Input: dimensioned drawing with shaded views. Units: mm. Origin: part minimum x, y, z. A direction names the side the tool comes from. Round coordinates to 2 decimals unless told otherwise and drop trailing zeros. Loops run counter-clockwise (first coordinate to the right, second up) from the corner with the lowest first, then second, coordinate; pieces in that order, holes last. Notation, with made-up numbers: (3, 64.25) - (36, 64.25) arc R14 cw to (36, 89.25) - close; hole circle Ø8 at (58, 24.25). An arc over 180 degrees is marked (long way). Answer as CSV lines item,"result".
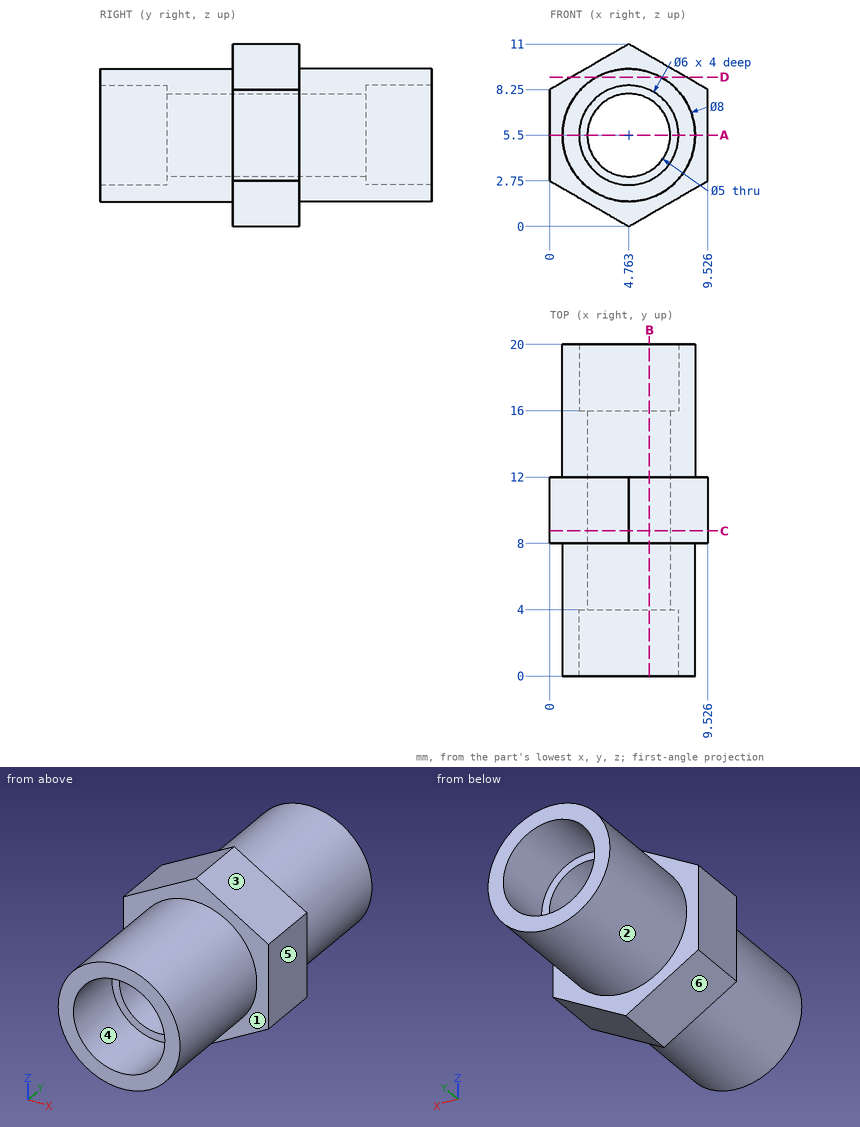
(1) Section A-A (z = 5.5). Output: boundary loops of the cut face in (x, y).
Findings below:
outline,"(0, 8) - (0.76, 8) - (0.76, 0) - (1.76, 0) - (1.76, 4) - (2.26, 4) - (2.26, 16) - (1.76, 16) - (1.76, 20) - (0.76, 20) - (0.76, 12) - (0, 12) - close; (7.26, 4) - (7.76, 4) - (7.76, 0) - (8.76, 0) - (8.76, 8) - (9.53, 8) - (9.53, 12) - (8.76, 12) - (8.76, 20) - (7.76, 20) - (7.76, 16) - (7.26, 16) - close"
(2) Section D-D (z = 9). Output: boundary loops of the cut face in (x, y).
Findings below:
outline,"(1.3, 8) - (2.83, 8) - (2.83, 0) - (6.7, 0) - (6.7, 8) - (8.23, 8) - (8.23, 12) - (6.7, 12) - (6.7, 20) - (2.83, 20) - (2.83, 12) - (1.3, 12) - close"
(3) Section C-C (y = 8.75). Output: boundary loops of the cut face in (x, z).
Findings below:
outline,"(0, 2.75) - (4.76, 0) - (9.53, 2.75) - (9.53, 8.25) - (4.76, 11) - (0, 8.25) - close; hole circle Ø5 at (4.76, 5.5)"
(4) Draft query along Z for the marked faces 4, 5 and 6. Return one class per face: pulls with the +Z half, pulls with the -Z half, needs draft (parallel to the pull), parting line crosses it, or undercut.
Findings below:
face 4,"undercut"
face 5,"needs draft"
face 6,"pulls with the -Z half"
(5) Material intervals for line 1 along X through (y, z) = (17.2, 5.5); line 2 along Z through (x, y) = (7, 4.5) (1 decimal); line 3 along X through (y, z) = (18.25, 2.75) (1 decimal), sorted ascending.
Findings below:
line 1,"0.76 to 1.76, 7.76 to 8.76"
line 2,"2.2 to 4.4, 6.6 to 8.8"
line 3,"1.9 to 3.6, 6 to 7.7"
(6) Pin query (flat end, axial travel): P1, Ø1, axis at x = 2, y = 13.5, coming from the -Z side; P2, Ø3, axis at x = 6, z = 4.5, coming from the +Y side; P3, Ø1.5, axis at y = 6, z = 7.5, coming from the -X side; P4, Ø3, axis at y = 17.5, z = 2, coming from the -X side. Return the tip coordinate at first contact, or that it passes through.
Findings below:
P1,"z = 2.2"
P2,"y = 20"
P3,"x = 0.96"
P4,"x = 1.3"
(7) Section B-B (x = 6). Output: boundary loops of the cut face in (y, z).
Findings below:
outline,"(0, 1.7) - (8, 1.7) - (8, 0.71) - (12, 0.71) - (12, 1.7) - (20, 1.7) - (20, 2.77) - (16, 2.77) - (16, 3.33) - (4, 3.33) - (4, 2.77) - (0, 2.77) - close; (0, 8.23) - (4, 8.23) - (4, 7.67) - (16, 7.67) - (16, 8.23) - (20, 8.23) - (20, 9.3) - (12, 9.3) - (12, 10.29) - (8, 10.29) - (8, 9.3) - (0, 9.3) - close"
(8) Access query for the marked faces 1, 2 and 3. Directions: +Z, -Z, +X, -X, +Y, -Y. A direction counts if a zero-diameter tool reaches every point of the face in a straight line with its end or side. Return the directions, or none.
Findings below:
face 1,"-Y"
face 2,"+Y"
face 3,"+Z, +X, +Y, -Y"
